Here's how the part is built. I have some questions about the finished solid (model axes, mm). Face numbers are marked on the shaded views. A direction names the side the tool comes from. Round coordinates to 2 decimals unless told otherwise and drop trailing zeros. Loops run counter-clockwise (first coordinate to the right, second up) from the corner with the lowest first, then second, coordinate; pieces in that order, holes last. Notation, with made-up numbers: (71.5, -14.5) -> (81.5, -14.5) arc R25 cw to (81.5, 3.5) -> close; hole circle Ø8 at (0, -12.5). An arc over 180 degrees is marked (long way). Use one line per item in the form item = value. Start each with the question number.
Item 1: If we section it at D-D (y = 0): Write out the boundary of the cut face in (x, z).
Item 2: For the marked faces 4, 5 and 6, which set-ups out of +Z, -Z, +X, -X, +Y, -Y let a thin tool reach every point of the face, with its end or its side?
Item 3: If we section it at C-C (z = 1.4): Write out the boundary of the cut face in (x, y), then the cut area to 3 significant figures.
Item 4: If we section it at A-A (y = -3.25): Write out the boundary of the cut face in (x, z).
Item 5: If I drill on L1, parallel to X at y = -3, z = 0.8; L2, parallel to X at y = -0.75, z = 0.5; L3, parallel to Y at x = 14, z = 1.15, over which ranges is the centre line in solid material (lowest first)? Write a range as [from, to].
Item 6: If we section it at B-B (x = -14): Write out the boundary of the cut face in (y, z), then the cut area to 3 significant figures.
Item 7: Thinking about a two-plate mould opening in X: for the marked faces 1, 2 and 3, which applies, released by +X, released by -X, zero draft, split by the parting line, or undercut?
Item 8: I'm going to push a flat-ended pin straight in: pin 1 Ø0.9 at (x, z) = (-2.5, 1) entering from -Y. Where does the tip first touch, or does it pass through?
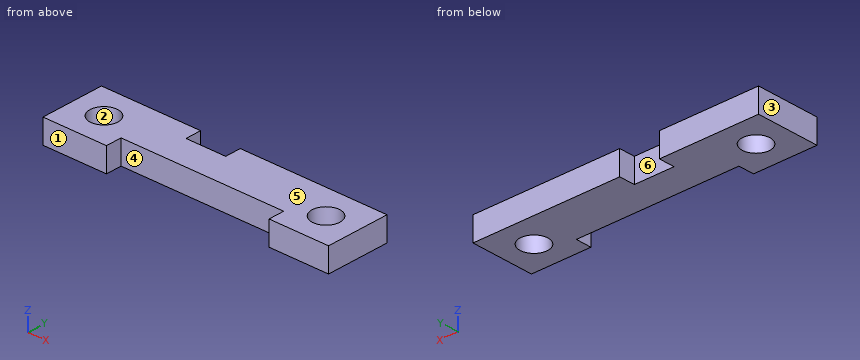
Autodesk Inventor part; units mm, degrees
ref_plane "YZ Plane" through (0, 0, 0) normal (1, 0, 0) x (0, 1, 0)
ref_plane "XZ Plane" through (0, 0, 0) normal (0, 1, 0) x (-1, 0, 0)
ref_plane "XY Plane" through (0, 0, 0) normal (0, 0, 1) x (1, 0, 0)
sketch "Sketch" plane through (0, 0, 0) normal (0, 0, 1) x (1, 0, 0)
  line L0 (-18, -4) -> (-18, 4)
  circle A0 centre (-14, 0) radius 1.75
  circle A1 centre (14, 0) radius 1.75
  line L1 (-10, -2) -> (-10, -4)
  line L2 (10.5, -2) -> (10.5, -4)
  line L3 (-18, -4) -> (-10, -4)
  line L4 (10.5, -4) -> (18, -4)
  line L5 (-5.5, 4) -> (-5.5, 2)
  line L6 (-5.5, 2) -> (-0.5, 2)
  line L7 (-0.5, 2) -> (-0.5, 4)
  line L8 (-0.5, 4) -> (5.8141, 4)
  line L9 (-0.5, 4) -> (18, 4)
  line L10 (18, 4) -> (18, -4)
  line L11 (-10, -2) -> (10.5, -2)
  line L12 (-5.5, 4) -> (-18, 4)
  line L13 (0, 15.191) -> (0, -14.809) construction
  point P0 (0, 0)
  point P1 (18, 0)
  dimension "d18" = 3.5
  dimension "d34" = 5
  dimension "d35" = 20.5
  dimension "d36" = 2
  dimension "d39" = 36
  dimension "d41" = 8
  dimension "d45" = 12.5
  dimension "d48" = 8
  dimension "d49" = 14
extrude "Extrusion" add sketch "Sketch" along normal blind 3
properties part number "solar_board_holder"
Values found:
q1.outline = (-18, 0) -> (-15.75, 0) -> (-15.75, 3) -> (-18, 3) -> close; (-12.25, 0) -> (12.25, 0) -> (12.25, 3) -> (-12.25, 3) -> close; (15.75, 0) -> (18, 0) -> (18, 3) -> (15.75, 3) -> close
q2.face_4 = +Z, -Z, -Y
q2.face_5 = +Z, +X, -X, +Y, -Y
q2.face_6 = +Z, -Z, +Y
q3.outline = (-18, -4) -> (-10, -4) -> (-10, -2) -> (10.5, -2) -> (10.5, -4) -> (18, -4) -> (18, 4) -> (-0.5, 4) -> (-0.5, 2) -> (-5.5, 2) -> (-5.5, 4) -> (-18, 4) -> close; hole circle Ø3.5 at (-14, 0); hole circle Ø3.5 at (14, 0)
q3.area = 218 mm2
q4.outline = (-18, 0) -> (-10, 0) -> (-10, 3) -> (-18, 3) -> close; (10.5, 0) -> (18, 0) -> (18, 3) -> (10.5, 3) -> close
q5.L1 = [-18, -10], [10.5, 18]
q5.L2 = [-18, -15.58], [-12.42, 12.42], [15.58, 18]
q5.L3 = [-4, -1.75], [1.75, 4]
q6.outline = (-4, 0) -> (-1.75, 0) -> (-1.75, 3) -> (-4, 3) -> close; (1.75, 0) -> (4, 0) -> (4, 3) -> (1.75, 3) -> close
q6.area = 13.5 mm2
q7.face_1 = zero draft
q7.face_2 = undercut
q7.face_3 = released by -X
q8.pin_1 = -2
